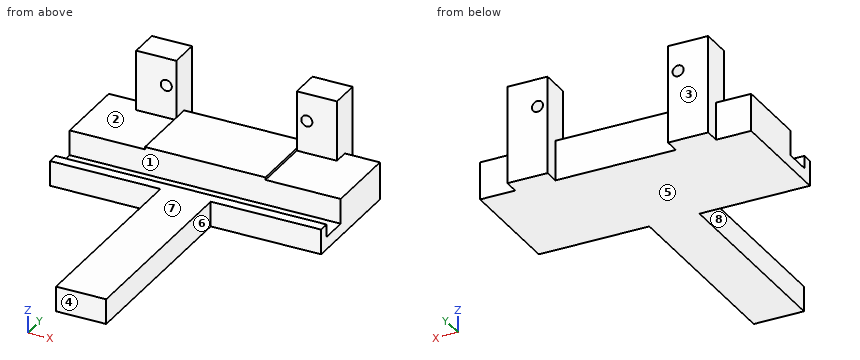
```python
from build123d import *

# Parameters (mm, degrees)
SKETCH_W        = 54
SKETCH_H        = 22.5
PAD_DEPTH       = 2.5
SKETCH001_W     = 54
SKETCH001_H     = 2.1
PAD001_DEPTH    = 2.5
SKETCH002_W     = 10
SKETCH002_H     = 5
PAD002_DEPTH    = 40
SKETCH003_W     = 54
SKETCH003_H     = 15
PAD003_DEPTH    = 5
SKETCH004_W     = 8
SKETCH004_H     = 3
PAD004_DEPTH    = 12
SKETCH005_R     = 1.1
POCKET_DEPTH    = 10
SKETCH006_W     = 8
SKETCH006_H     = 19.5
PAD005_DEPTH    = 3
SKETCH007_R     = 1.1
POCKET001_DEPTH = 5
SKETCH008_W     = 24
SKETCH008_H     = 15
PAD006_DEPTH    = 0.5


with BuildPart() as part:
    # Sketch → Pad (new body)
    with BuildSketch(Plane.XY):
        with Locations((0, -11.25)):
            Rectangle(SKETCH_W, SKETCH_H)
    extrude(amount=PAD_DEPTH)

    # Sketch001 (on Face6 of Pad) → Pad001 (join)
    with BuildSketch(Plane.XY.offset(2.5)):
        with Locations((0, -21.45)):
            Rectangle(SKETCH001_W, SKETCH001_H)
    extrude(amount=PAD001_DEPTH)

    # Sketch002 (on Face10 of Pad001) → Pad002 (join)
    with BuildSketch(Plane.XZ.offset(22.5)):
        with Locations((0, 2.5)):
            Rectangle(SKETCH002_W, SKETCH002_H)
    extrude(amount=PAD002_DEPTH)

    # Sketch003 (on Face5 of Pad002) → Pad003 (join)
    with BuildSketch(Plane.XY.offset(2.5)):
        with Locations((0, -7.5)):
            Rectangle(SKETCH003_W, SKETCH003_H)
    extrude(amount=PAD003_DEPTH)

    # Sketch004 (on Face14 of Pad003) → Pad004 (join)
    with BuildSketch(Plane.XY.offset(7.5)):
        with Locations((16, -1.5)):
            Rectangle(SKETCH004_W, SKETCH004_H)
        with Locations((-16, -1.5)):
            Rectangle(SKETCH004_W, SKETCH004_H)
    extrude(amount=PAD004_DEPTH)

    # Sketch005 (on Face26 of Pad004) → Pocket (cut)
    with BuildSketch(Plane.XZ.offset(3)):
        with Locations((-14, 14)):
            Circle(SKETCH005_R)
        with Locations((14, 14)):
            Circle(SKETCH005_R)
    extrude(amount=-POCKET_DEPTH, mode=Mode.SUBTRACT)

    # Sketch006 (on Face5 of Pocket) → Pad005 (join)
    with BuildSketch(Plane(origin=(0, 0, 0), x_dir=(-1, 0, 0), z_dir=(0, 1, 0))):
        with Locations((-16, 9.75)):
            Rectangle(SKETCH006_W, SKETCH006_H)
        with Locations((16, 9.75)):
            Rectangle(SKETCH006_W, SKETCH006_H)
    extrude(amount=PAD005_DEPTH)

    # Sketch007 (on Face49 of Pad005) → Pocket001 (cut)
    with BuildSketch(Plane.XZ):
        with Locations((-14, 14)):
            Circle(SKETCH007_R)
        with Locations((14, 14)):
            Circle(SKETCH007_R)
    extrude(amount=-POCKET001_DEPTH, mode=Mode.SUBTRACT)

    # Sketch008 (on Face17 of Pocket001) → Pad006 (join)
    with BuildSketch(Plane.XY.offset(7.5)):
        with Locations((0, -7.5)):
            Rectangle(SKETCH008_W, SKETCH008_H)
    extrude(amount=PAD006_DEPTH)


solid = part.part
```
Geometry check sheet. Reference: the model listing, model coordinates, mm. Face numbers are marked on the shaded views. A direction names the side the tool comes from. Give positions to 0.01 mm unless a question says otherwise; leave off trailing zeros. Loops run counter-clockwise (first coordinate to the right, second up) from the corner with the lowest first, then second, coordinate; pieces in that order, holes last. Notation, with made-up numbers: (75.5, -32) - (134.5, -32) arc R10 ccw to (134.5, -22) - close; hole circle Ø11 at (66.25, 62.5). An arc over 180 degrees is marked (long way). Use CSV: the item, a comma, the result in double quotes. Start each with the question number.
Q1. Section check B-B, the plane x = -14. Record the cut outline in (y, z).
Q2. Section check D-D, the plane x = 18. Record the cut outline in (y, z), and give its area (3 significant figures).
Q3. Release check for a two-part mould opening along Y. For the marked faces 1, 2 and 3 record: +Y half, -Y half, draft (parallel to the pull), parting line (faces both ways), or undercut.
Q4. Section check C-C, the plane z = 6. Record the cut outline in (x, y).
Q5. Scan lines: probe 1 along Z at (x, y) = (14, -1); probe 2 along Z at (x, y) = (2.5, -18); probe 3 along Y at (x, z) = (7, 1.75). Record each from-to range of solid material in increasing order. Write a range as from..to.
Q6. Section check A-A, the plane z = 10.5. Record the cut outline in (x, y).
Q7. Go/stop test with flat-tipped pins: pin 1 Ø1.6 at (x, z) = (-12.5, 5) entering from -Y; pin 2 Ø2 at (x, z) = (-22, 3) entering from +Y; pin 3 Ø3 at (y, z) = (-56, 3.5) entering from +X. Record where each tip stops, or that it passes through.
Q8. Access from +Z, -Z, +X, -X, +Y, -Y to the whole of each face (thin tool, end or side, straight path). Record for the marked faces 4, 5, 6, 7 and 8.
Findings below:
1,outline,"(-22.5, 0) - (3, 0) - (3, 12.9) - (-3, 12.9) - (-3, 7.5) - (-15, 7.5) - (-15, 2.5) - (-20.4, 2.5) - (-20.4, 5) - (-22.5, 5) - close; (-3, 15.1) - (3, 15.1) - (3, 19.5) - (-3, 19.5) - close"
2,outline,"(-22.5, 0) - (3, 0) - (3, 19.5) - (-3, 19.5) - (-3, 7.5) - (-15, 7.5) - (-15, 2.5) - (-20.4, 2.5) - (-20.4, 5) - (-22.5, 5) - close"
2,area,"231 mm^2"
3,face 1,"undercut"
3,face 2,"draft"
3,face 3,"+Y half"
4,outline,"(-27, -15) - (27, -15) - (27, 0) - (20, 0) - (20, 3) - (12, 3) - (12, 0) - (-12, 0) - (-12, 3) - (-20, 3) - (-20, 0) - (-27, 0) - close"
5,probe 1,"z = 0..12.9, 15.1..19.5"
5,probe 2,"z = 0..2.5"
5,probe 3,"y = -22.5..0"
6,outline,"(-20, -3) - (-12, -3) - (-12, 3) - (-20, 3) - close; (12, -3) - (20, -3) - (20, 3) - (12, 3) - close"
7,pin 1,"stops at y = -22.5"
7,pin 2,"stops at y = 0"
7,pin 3,"stops at x = 5"
8,face 4,"+Z, -Z, +X, -X, -Y"
8,face 5,"-Z, +X, -X, +Y, -Y"
8,face 6,"+Z, -Z, +X, -Y"
8,face 7,"+Z, +X, -X, -Y"
8,face 8,"+Z, -Z, -X, -Y"
